```python
from build123d import *

# Parameters (mm, degrees)
PAD_DEPTH       = 20
SKETCH001_R     = 8
POCKET_DEPTH    = 5
SKETCH002_R     = 5
POCKET001_DEPTH = 5


with BuildPart() as part:
    # Sketch → Pad (new body)
    with BuildSketch(Plane.XY):
        with BuildLine():
            Line((60, 8), (60, 82.000001))
            ThreePointArc((60, 82.000001), (58.434586, 89.869877), (53.976662, 96.541638))
            Line((40.541631, 109.976664), (53.976662, 96.541638))
            ThreePointArc((40.541631, 109.976664), (33.869872, 114.434584), (25.999999, 115.999997))
            Line((7.999999, 115.999997), (25.999999, 115.999997))
            ThreePointArc((7.999999, 115.999997), (2.343146, 113.656851), (0, 107.999998))
            Line((0, 107.999998), (0, 8))
            ThreePointArc((0, 8), (2.343146, 2.343146), (8, 0))
            Line((8, 0), (52, 0))
            ThreePointArc((52, 0), (57.656854, 2.343146), (60, 8))
        make_face()
        with BuildLine():
            ThreePointArc((8.00002, 113.999997), (3.757366, 112.242645), (2, 107.999998))
            Line((2, 107.999998), (2, 8))
            ThreePointArc((2, 8), (3.757359, 3.757359), (8, 2))
            Line((8, 2), (52, 2))
            ThreePointArc((52, 2), (56.242641, 3.757359), (58, 8))
            Line((58, 82), (58, 8))
            ThreePointArc((58, 82), (56.586824, 89.104516), (52.562438, 95.127434))
            Line((39.127428, 108.56244), (52.562438, 95.127434))
            ThreePointArc((39.127428, 108.56244), (33.104513, 112.586822), (25.999999, 113.999997))
            Line((8.00002, 113.999997), (25.999999, 113.999997))
        make_face(mode=Mode.SUBTRACT)
    extrude(amount=PAD_DEPTH)

    # Sketch001 → Pocket (cut)
    with BuildSketch(Plane(origin=(75.259141, 75.259166, 0), x_dir=(-0.707107, 0.707107, 0), z_dir=(0.707107, 0.707107, 0))):
        with Locations((39.5, 10)):
            Circle(SKETCH001_R)
    extrude(amount=-POCKET_DEPTH, mode=Mode.SUBTRACT)

    # Sketch002 → Pocket001 (cut)
    with BuildSketch(Plane(origin=(0, 115.999997, 0), x_dir=(-1, 0, 0), z_dir=(0, 1, 0))):
        with Locations((-17, 10)):
            Circle(SKETCH002_R)
    extrude(amount=-POCKET001_DEPTH, mode=Mode.SUBTRACT)


solid = part.part
```
Verification items for the finished model (mm, model axes). A direction names the side the tool comes from. Give positions to 0.01 mm unless a question says otherwise; leave off trailing zeros. Order: outer loops, then holes, each group sorted by start corner. A loop starts at its lowest first (then second) coordinate and runs counter-clockwise, first axis right, second up. Notation, with made-up numbers: M 11.5,69.5 L 39.5,69.5 A23 cw 39.5,100.5 Z; hole C 5.5,48.25 d7. An arc over 180 degrees is marked long. Return JSON: item names as keys, results as strings. Group by question number.
1) Section check B-B on x = 10. Record the cut outline in (y, z).
2) Section check D-D on x = 17. Record the cut outline in (y, z).
3) Section check C-C on z = 10. Record the cut outline in (x, y) (3 decimals).
4) Access from +Z, -Z, +X, -X, +Y, -Y to the whole of each face (thin tool, end or side, straight path). Record for faces 5 (the face through (3.711, 3.804, 9.86)), 6 (the face through (1, 67, 0)).
5) Mould release check, pull along X, two halves, no side actions. Record for faces 1 (the face through (30, 0, 10)), 2 (the face through (15, 114, 5)), 3 (the face through (2.281, 2.406, 9.86)), 4 (the face through (3.804, 112.289, 9.86)): pulls with the +X half, pulls with the -X half, needs draft (parallel to the pull), parting line crosses it, or undercut.
6) Go/stop test with flat-tipped pins: pin 1 Ø1.5 at (y, z) = (98, 16) entering from +X; pin 2 Ø5 at (x, z) = (32.5, 9) entering from +Y; pin 3 Ø6 at (x, z) = (35, 9) entering from +Y. Record where each tip stops, or that it passes through.
7) Scan lines: line 1 (Z direction, x = 17, y = 114.7); line 2 (X direction, y = 54, z = 10); line 3 (Y direction, x = 22.5, z = 12). Record each from-to range of solid material in increasing order.
8) Section check A-A on y = 59. Record the cut outline in (x, z).
Answer block:
{
 "1": {"outline": "M 0,0 L 2,0 L 2,20 L 0,20 Z; M 114,0 L 116,0 L 116,20 L 114,20 Z"},
 "2": {"outline": "M 0,0 L 2,0 L 2,20 L 0,20 Z; M 114,0 L 116,0 L 116,5 L 114,5 Z; M 114,15 L 116,15 L 116,20 L 114,20 Z"},
 "3": {"outline": "M 0,8 A8 ccw 8,0 L 52,0 A8 ccw 60,8 L 60,82 A20.565 ccw 53.977,96.542 L 52.985,97.533 L 51.571,96.119 L 52.562,95.127 A18.565 cw 58,82 L 58,8 A6 cw 52,2 L 8,2 A6 cw 2,8 L 2,108 A6 cw 8,114 L 12,114 L 12,116 L 8,116 A8 ccw 0,108 Z; M 22,114 L 26,114 A18.565 cw 39.127,108.562 L 40.257,107.433 L 41.672,108.847 L 40.542,109.977 A20.565 ccw 26,116 L 22,116 Z"},
 "4": {"face 5": "+Z, -Z", "face 6": "-Z, +X, -X, +Y, -Y"},
 "5": {"face 1": "needs draft", "face 2": "undercut", "face 3": "pulls with the -X half", "face 4": "undercut"},
 "6": {"pin 1": "stops at x = 53.27", "pin 2": "stops at y = 115.61", "pin 3": "stops at y = 115.11"},
 "7": {"line 1": "z = 0 to 5, 15 to 20", "line 2": "x = 0 to 2, 58 to 60", "line 3": "y = 0 to 2, 114 to 116"},
 "8": {"outline": "M 0,0 L 2,0 L 2,20 L 0,20 Z; M 58,0 L 60,0 L 60,20 L 58,20 Z"}
}
